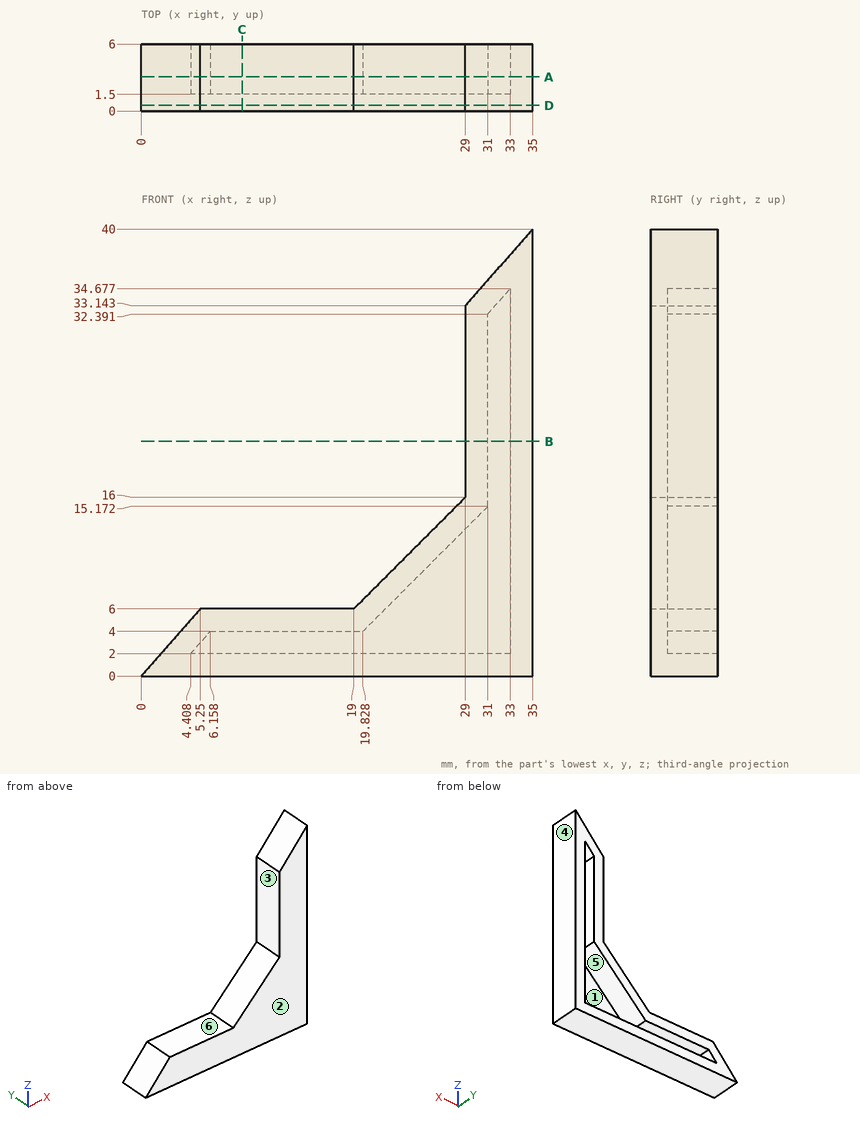
Print and shaded views of the part. All mm, measured from the part's lowest x, y and z. A direction names the side the tool comes from. Coordinates: 2 decimals unless noted, no trailing zeros. Order: outer loops, then holes, each group sorted by start corner. A loop starts at its lowest first (then second) coordinate and runs counter-clockwise, first axis right, second up. Notation, with made-up numbers: (18, -34) - (45, -34) arc R18 cw to (45, -28) - close; hole circle Ø9 at (72.25, 20). An arc over 180 degrees is marked (long way). Put each result on its own line as item: value.
1. Pull direction Z, two halves, no side cores. Call the marked faces 4, 5 and 6: pulls with the +Z half, pulls with the -Z half, needs draft (parallel to the pull), parting line crosses it, or undercut.
Answer sheet:
face 4: needs draft
face 5: undercut
face 6: pulls with the +Z half
2. Tool access for the marked faces 1, 2 and 3: list every direction of +Z, -Z, +X, -X, +Y, -Y with a clear straight run to the whole face (end or side of a thin tool).
Answer sheet:
face 1: +Y
face 2: +Z, -Z, +X, -X, -Y
face 3: +Z, -X, +Y, -Y
3. Saw through at B-B (z = 21). Write the cut outline in (x, y).
Answer sheet:
outline: (29, 0) - (35, 0) - (35, 6) - (33, 6) - (33, 1.5) - (31, 1.5) - (31, 6) - (29, 6) - close
4. Probe line 1 along Z through (x, y) = (17, 3.45); line 2 along X through (y, z) = (4.4, 18.5); line 3 along X through (y, z) = (0.55, 16). List the from-to ranges inside material, lowest first. Write a range as [from, to].
Answer sheet:
line 1: z = [0, 2], [4, 6]
line 2: x = [29, 31], [33, 35]
line 3: x = [29, 35]
5. Drop flat-ended pins along their axis: P1, Ø3, axis at x = 24, y = 5, coming from the +Z side; P2, Ø2, axis at y = 5, z = 12, coming from the -X side; P3, Ø3, axis at x = 28, z = 7, coming from the +Y side. Give the stop position or say it passes through.
Answer sheet:
P1: stops at z = 12.5
P2: stops at x = 24
P3: stops at y = 1.5
6. Saw through at A-A (y = 3.05). Write the cut outline in (x, z).
Answer sheet:
outline: (0, 0) - (35, 0) - (35, 40) - (29, 33.14) - (29, 16) - (19, 6) - (5.25, 6) - close; hole (4.41, 2) - (33, 2) - (33, 34.68) - (31, 32.39) - (31, 15.17) - (19.83, 4) - (6.16, 4) - close
7. Saw through at D-D (y = 0.5). Write the cut outline in (x, z), and give its area (3 significant figures).
Answer sheet:
outline: (0, 0) - (35, 0) - (35, 40) - (29, 33.14) - (29, 16) - (19, 6) - (5.25, 6) - close
area: 428 mm^2
8. Saw through at C-C (x = 9). Write the cut outline in (y, z).
Answer sheet:
outline: (0, 0) - (6, 0) - (6, 2) - (1.5, 2) - (1.5, 4) - (6, 4) - (6, 6) - (0, 6) - close
